Geometry: final body of the model. Coordinates: model frame, mm. A direction names the side the tool comes from. Coordinates: 2 decimals unless noted, no trailing zeros. Loops run counter-clockwise (first coordinate to the right, second up) from the corner with the lowest first, then second, coordinate; pieces in that order, holes last. Notation, with made-up numbers: (-6.75, -13.75) - (28.25, -13.75) arc R20 cw to (28.25, -6.75) - close; hole circle Ø5 at (84.5, 11.5). An arc over 180 degrees is marked (long way). Put each result on its own line as item: value. Start each with the question number.
1) Section A-A on z = 1.25. Output: boundary loops of the cut face in (x, y).
2) Section D-D on y = 12. Output: boundary loops of the cut face in (x, z).
3) Reachability of faces 1 (the flat face through (-4, -31, 7)), 2 (the flat face through (-1, 1, -3)) from +Z, -Z, +X, -X, +Y, -Y: full face, straight path, thin tool, end or side. Return the list, or none.
4) Material intervals for line 1 along Y through (x, z) = (22.5, 10); line 2 along Y through (x, z) = (-16, 1); line 3 along Y through (x, z) = (-14.5, 3.25), sorted ascending. Write a range as from..to.
5) Draft query along Y for faces 3 (the flat face through (-1, 40, 1)), 4 (the flat face through (18, -30, 1)), 5 (the flat face through (0, 0, 11)). Return one class per face: +Y half, -Y half, draft (parallel to the pull), parting line (faces both ways), or undercut.
6) Contact query for flat-ended pins moving along their axis: pin 1 Ø5 at (x, z) = (-3, 9) entering from -Y; pin 2 Ø1.5 at (y, z) = (23.5, 7.5) entering from +X; pin 3 Ø6.5 at (y, z) = (-14.5, 7) entering from +X; pin 4 Ø2.5 at (y, z) = (-10, 7.5) entering from -X. Output: stop coordinate, or through.
7) Section B-B on x = 3. Output: boundary loops of the cut face in (y, z).
```python
from build123d import *

# Parameters (mm, degrees)
F1_START = 3
F0_W     = 80
F0_H     = 80
F0_W_2   = 76
F0_H_2   = 76
F1_DEPTH = 51
F0_W_3   = 70
F0_H_3   = 70
F2_DEPTH = 3
F4_W     = 60
F4_H     = 60
F5_DEPTH = 3
F7_DEPTH = 5
F9_DEPTH = 11


# Not quite as in the source:
# - a pattern or mirror of a feature is missing from the dataset's text; its kind, count and spacing are read off the source's solid


with BuildPart() as f1:
    # F0 (on Top) → F1 (new body)
    with BuildSketch(Plane.XY.offset(F1_START)):
        Rectangle(F0_W, F0_H)
        Rectangle(F0_W_2, F0_H_2, mode=Mode.SUBTRACT)
    extrude(amount=F1_DEPTH)


with BuildPart() as f2:
    # F0 (on Top) → F2 (new body)
    with BuildSketch(Plane.XY):
        Rectangle(F0_W, F0_H)
        Rectangle(F0_W_2, F0_H_2, mode=Mode.SUBTRACT)
        Rectangle(F0_W_2, F0_H_2)
        Rectangle(F0_W_3, F0_H_3, mode=Mode.SUBTRACT)
        Rectangle(F0_W_3, F0_H_3)
    extrude(amount=-F2_DEPTH)

    # F4 (on Top) → F5 (join)
    with BuildSketch(Plane.XY):
        Rectangle(F4_W, F4_H)
    extrude(amount=F5_DEPTH)

    # F0 (on Top) → F7 (join)
    with BuildSketch(Plane.XY):
        Rectangle(F0_W, F0_H)
        Rectangle(F0_W_2, F0_H_2, mode=Mode.SUBTRACT)
    extrude(amount=F7_DEPTH)

    # F8 (on Top) → F9 (join)
    with BuildSketch(Plane.XY):
        Polygon((-35, 0), (35, 0), (35, 5), (6, 5), (6, 8), (26, 8), (26, 26), (9, 26), (9, 15), (6, 15), (6, 35), (-4, 35), (-4, 26), (-25, 26), (-25, 8), (-7, 8), (-7, 19), (-4, 19), (-4, 5), (-35, 5), align=None)
    f9 = extrude(amount=F9_DEPTH)

    # F9_copies: F9 across plane
    add(f9.mirror(Plane(origin=(0, 0, 0), x_dir=(0, 0, -1), z_dir=(0, -1, 0))))


solid = f2.part
```
Answer block:
1. outline: (-40, -40) - (40, -40) - (40, 40) - (-40, 40) - close; (-35, -5) - (-30, -5) - (-30, -30) - (-4, -30) - (-4, -35) - (6, -35) - (6, -30) - (30, -30) - (30, -5) - (35, -5) - (35, 5) - (30, 5) - (30, 30) - (6, 30) - (6, 35) - (-4, 35) - (-4, 30) - (-30, 30) - (-30, 5) - (-35, 5) - close; hole (-38, -38) - (38, -38) - (38, 38) - (-38, 38) - close
2. outline: (-40, -3) - (40, -3) - (40, 5) - (38, 5) - (38, 0) - (30, 0) - (30, 3) - (26, 3) - (26, 11) - (-4, 11) - (-4, 3) - (-7, 3) - (-7, 11) - (-25, 11) - (-25, 3) - (-30, 3) - (-30, 0) - (-38, 0) - (-38, 5) - (-40, 5) - close
3. face 1: +Z
3. face 2: -Z, +X, -X, +Y, -Y
4. line 1: y = -26..-8, -5..5, 8..26
4. line 2: y = -40..-38, -30..30, 38..40
4. line 3: y = -40..-38, -26..-8, -5..5, 8..26, 38..40
5. face 3: +Y half
5. face 4: undercut
5. face 5: draft
6. pin 1: stops at y = -35
6. pin 2: stops at x = 26
6. pin 3: stops at x = 40
6. pin 4: stops at x = -25
7. outline: (-40, -3) - (40, -3) - (40, 5) - (38, 5) - (38, 0) - (35, 0) - (35, 11) - (-35, 11) - (-35, 0) - (-38, 0) - (-38, 5) - (-40, 5) - close
